Can you work these out from the drawing? Everything is in mm from the part's minimum corner. Coordinates: 2 decimals unless noted, no trailing zeros. Order: outer loops, then holes, each group sorted by start corner. A loop starts at its lowest first (then second) coordinate and runs counter-clockwise, first axis right, second up. Notation, with made-up numbers: (28, 40.25) - (85, 40.25) arc R24 cw to (85, 50.25) - close; hole circle Ø6 at (18, 42.25). An arc over 180 degrees is marked (long way). One line per item, written item: value.
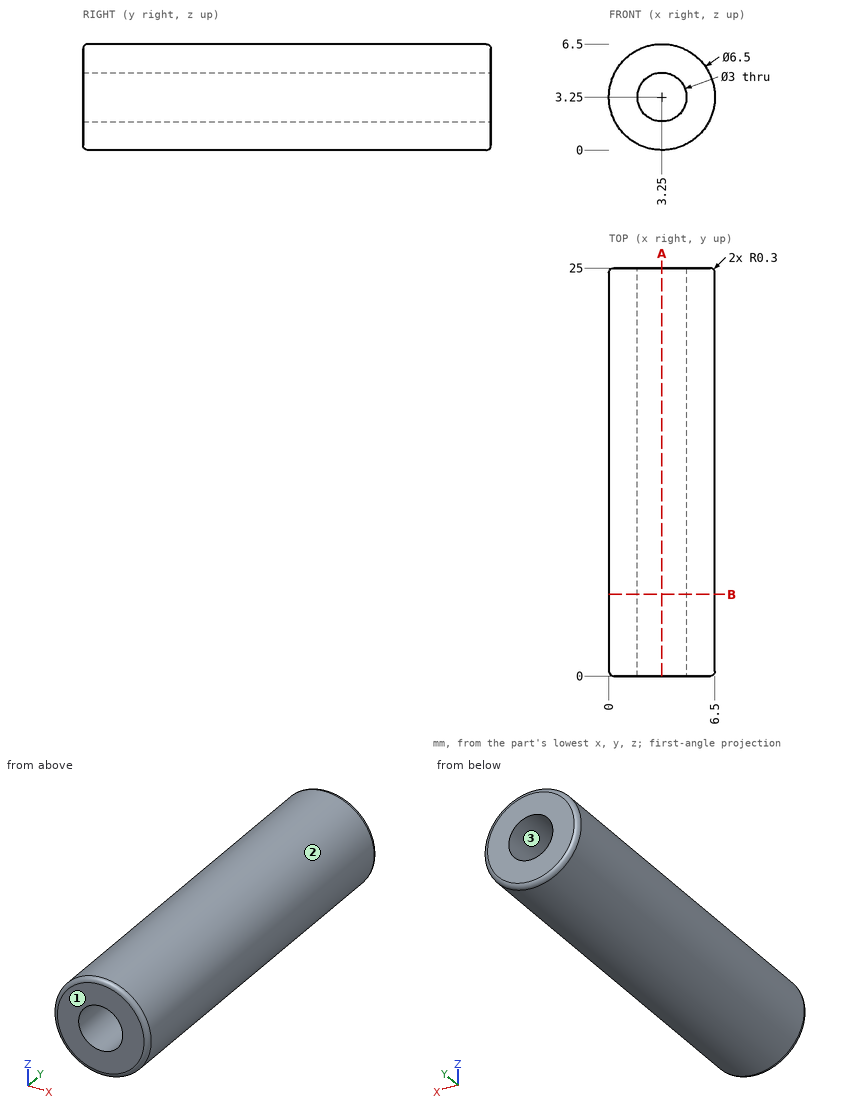
Item 1: I'm going to push flat-ended pins straight in: pin 1 Ø3 at (y, z) = (13, 1.5) entering from -X; pin 2 Ø2.5 at (x, z) = (3.25, 3.25) entering from -Y; pin 3 Ø1 at (y, z) = (8.5, 1.5) entering from -X; pin 4 Ø3 at (x, y) = (5, 15) entering from -Z. Where does each tip first touch, or does it pass through?
Conclusion:
pin 1: x = 0.01
pin 2: through
pin 3: x = 0.25
pin 4: z = 0.01
Item 2: I want a section at B-B on y = 5. Please give me the cut outline in (x, z).
Conclusion:
outline: circle Ø6.5 at (3.25, 3.25); hole circle Ø3 at (3.25, 3.25)
Item 3: I want a section at A-A on x = 3.25. Please give me the cut outline in (y, z).
Conclusion:
outline: (0, 0.3) arc R0.3 ccw to (0.3, 0) - (24.7, 0) arc R0.3 ccw to (25, 0.3) - (25, 1.75) - (0, 1.75) - close; (0, 4.75) - (25, 4.75) - (25, 6.2) arc R0.3 ccw to (24.7, 6.5) - (0.3, 6.5) arc R0.3 ccw to (0, 6.2) - close
Item 4: If I drill on probe 1 along Z at (x, y) = (3.25, 9.75); probe 2 along X at (y, z) = (22.75, 2.5); probe 3 along X at (y, z) = (11, 3.5), over which ranges is the centre line in solid material (lowest first)?
Conclusion:
probe 1: 0 to 1.75, 4.75 to 6.5
probe 2: 0.09 to 1.95, 4.55 to 6.41
probe 3: 0.01 to 1.77, 4.73 to 6.49
Item 5: Thinking about a two-plate mould opening in X: for the marked faces 1, 2 and 3, which applies, pulls with the +X half, pulls with the -X half, needs draft (parallel to the pull), parting line crosses it, or undercut?
Conclusion:
face 1: needs draft
face 2: parting line crosses it
face 3: undercut
